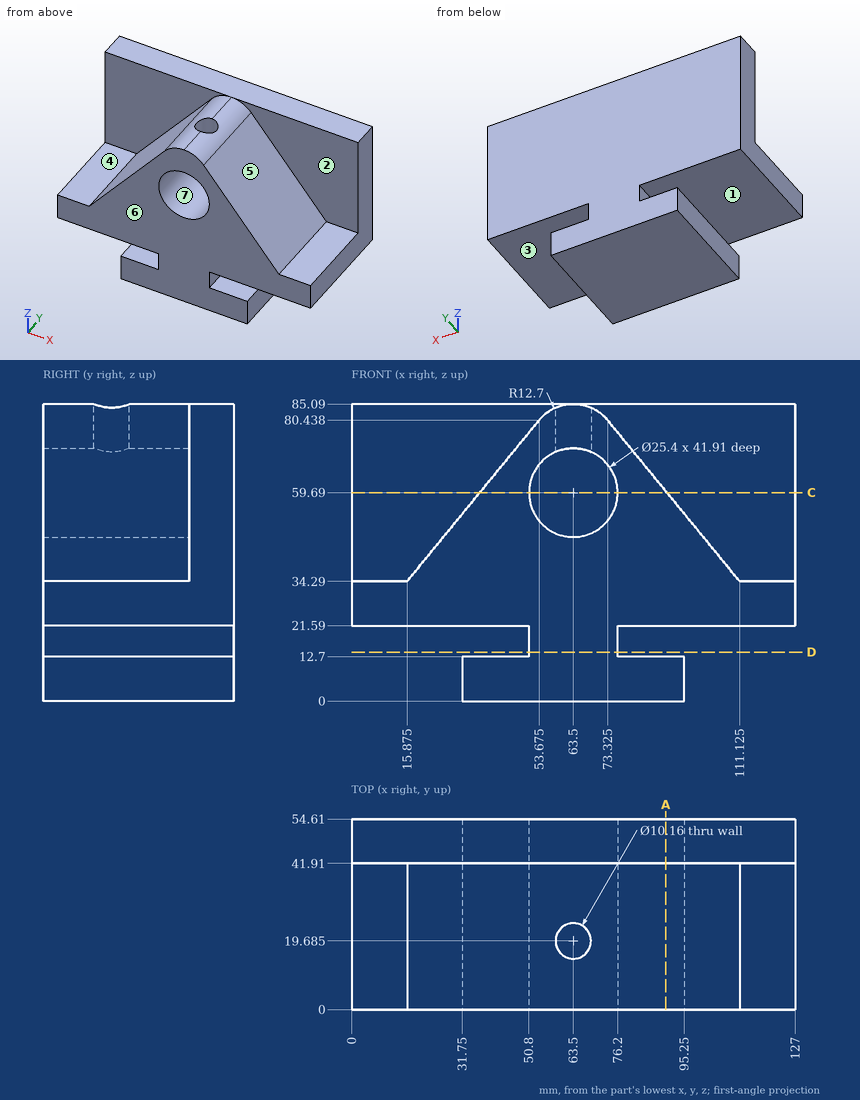
Verification items for this drawing (mm, ordinates from the low corner). A direction names the side the tool comes from. Coordinates: 2 decimals unless noted, no trailing zeros. Order: outer loops, then holes, each group sorted by start corner. A loop starts at its lowest first (then second) coordinate and runs counter-clockwise, first axis right, second up. Notation, with made-up numbers: (-21.5, 34) - (26.5, 34) arc R21 ccw to (26.5, 49) - close; hole circle Ø8 at (25, 26). An arc over 180 degrees is marked (long way). Answer in a Markdown table with one row per item. Add a question column.
1. Section check C-C (z = 59.69). Enter the section's corners in (x, y), plus the area to 3 significant figures.
2. Section check D-D (z = 14). Enter the section's corners in (x, y), plus the area to 3 significant figures.
3. Material ranges on L1, parallel to Y at x = 63.5, z = 78 (1 decimal); L2, parallel to Z at x = 63, y = 28; L3, parallel to Y at x = 119, z = 38, recorded low to high. Write a range as [from, to].
4. Section check A-A (x = 90). Enter the section's corners in (y, z), plus the area to 3 significant figures.
5. Gauge pin test, flat ends, axial feed: pin 1 Ø10 at (y, z) = (38, 4.5) entering from +X; pin 2 Ø12 at (x, y) = (13, 28) entering from -Z; pin 3 Ø17.5 at (x, y) = (4, 12) entering from +Z; pin 4 Ø8 at (y, z) = (33, 36) entering from +X. Record the tip position at first contact, or that the pin passes through.
6. Draft check along Z on the marked faces 5, 6 and 7. Enter one of: +Z half, -Z half, draft (parallel to the pull), parting line (faces both ways), or undercut.
7. Access from +Z, -Z, +X, -X, +Y, -Y to the whole of each face (thin tool, end or side, straight path). Record for the marked faces 1, 2, 3 and 4.
Data:
| question | item | result |
|---|---|---|
| 1 | outline | (0, 41.91) - (36.68, 41.91) - (36.68, 0) - (50.8, 0) - (50.8, 41.91) - (76.2, 41.91) - (76.2, 0) - (90.32, 0) - (90.32, 41.91) - (127, 41.91) - (127, 54.61) - (0, 54.61) - close |
| 1 | area | 2,800 mm² |
| 2 | outline | (50.8, 0) - (76.2, 0) - (76.2, 54.61) - (50.8, 54.61) - close |
| 2 | area | 1,390 mm² |
| 3 | L1 | y = [0, 14.6], [24.8, 54.6] |
| 3 | L2 | z = [0, 47], [72.38, 85.08] |
| 3 | L3 | y = [41.91, 54.61] |
| 4 | outline | (0, 0) - (54.61, 0) - (54.61, 12.7) - (0, 12.7) - close; (0, 21.59) - (54.61, 21.59) - (54.61, 85.09) - (41.91, 85.09) - (41.91, 60.08) - (0, 60.08) - close |
| 4 | area | 3,110 mm² |
| 5 | pin 1 | stops at x = 95.25 |
| 5 | pin 2 | stops at z = 21.59 |
| 5 | pin 3 | stops at z = 34.29 |
| 5 | pin 4 | stops at x = 127 |
| 6 | face 5 | +Z half |
| 6 | face 6 | draft |
| 6 | face 7 | undercut |
| 7 | face 1 | -X, +Y, -Y |
| 7 | face 2 | +Z, +X, -Y |
| 7 | face 3 | +X, +Y, -Y |
| 7 | face 4 | +Z, -X, -Y |
